Geometry check sheet. Reference: drawing and pictorial views, mm from the part's lowest x, y, z. Give positions to 0.01 mm unless a question says otherwise; leave off trailing zeros. Write each loop counter-clockwise with the first axis right and the second up, starting at its lowest first coordinate (ties: lowest second). Pieces come first, ordered by that corner, then holes. Notation, with made-up numbers: (-29, 31) - (-21, 31) arc R24 ccw to (-21, 44) - close; hole circle Ø1 at (70, 64). An arc over 180 degrees is marked (long way). Write item = value, one per line. Start each with the question number.
(1) Section check A-A, the plane y = 3. Enter the section's corners in (x, z), plus the area to 3 significant figures.
(2) Depth check by flat-ended pin: pin 1 Ø1.5 at (x, y) = (3, 2) entering from -Z; pin 2 Ø1.5 at (y, z) = (2.5, 151.5) entering from -X; pin 3 Ø2.5 at (y, z) = (2, 3) entering from +X; pin 4 Ø1 at (y, z) = (2.5, 136) entering from -X. Enter the tip coordinate at first touch or a pass-through.
(3) Section check B-B, the plane x = 5. Enter the section's corners in (y, z).
(4) Thickness scan on L1, parallel to Z at x = 26, y = 3.8. Record the ranges inside material, lowest first.
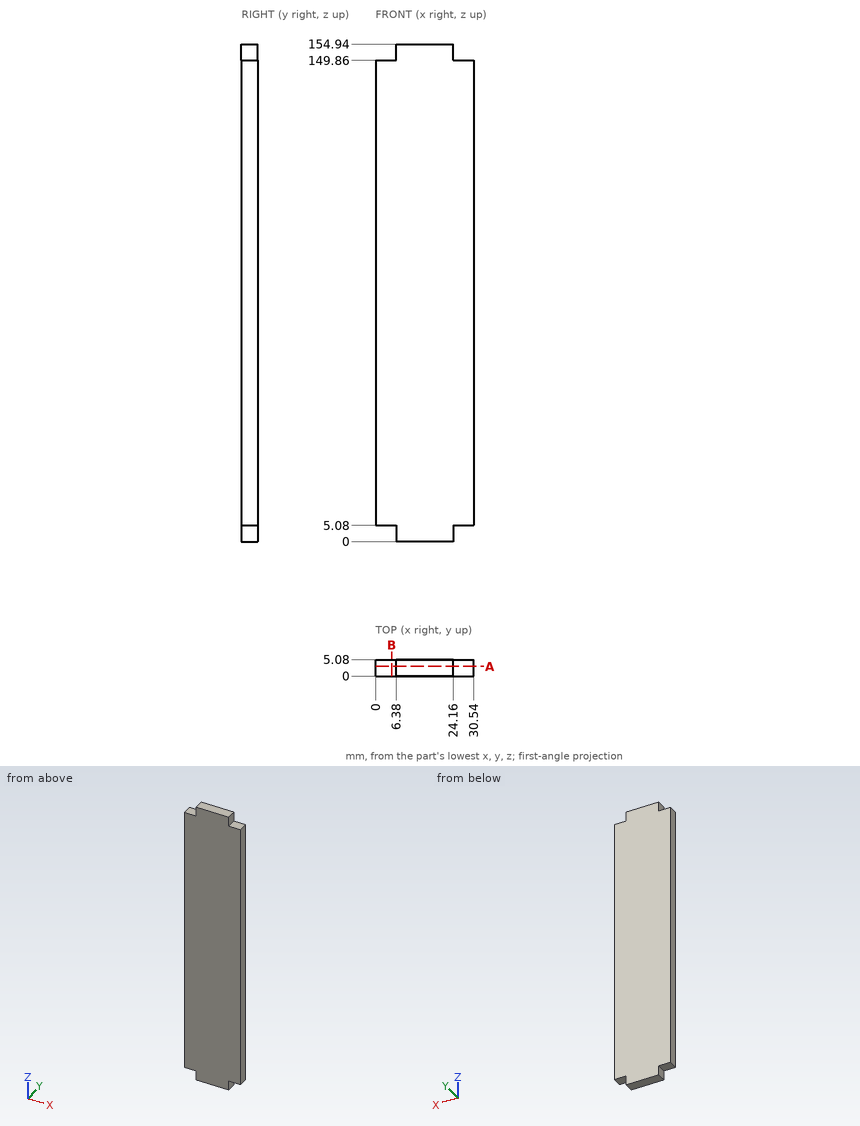
Model answer:
q1.outline = (0, 5.08) - (6.38, 5.08) - (6.38, 0) - (24.16, 0) - (24.16, 5.08) - (30.54, 5.08) - (30.54, 149.86) - (24.16, 149.86) - (24.16, 154.94) - (6.38, 154.94) - (6.38, 149.86) - (0, 149.86) - close
q1.area = 4,600 mm²
q2.pin_1 = 5.08
q2.pin_2 = 6.38
q2.pin_3 = 24.16
q2.pin_4 = 0
q3.outline = (0, 5.08) - (5.08, 5.08) - (5.08, 149.86) - (0, 149.86) - close
q4.L1 = 5.08 to 149.86
